Check sheet for the modelled part. Datum: model origin and axes. Units: mm. Give positions to 0.01 mm unless a question says otherwise; leave off trailing zeros. Loops run counter-clockwise (first coordinate to the right, second up) from the corner with the lowest first, then second, coordinate; pieces in that order, holes last. Notation, with made-up numbers: (51.5, 28.5) -> (77.5, 28.5) arc R17 cw to (77.5, 45.5) -> close; hole circle Ø8 at (-20.75, -0.75). An arc over 180 degrees is marked (long way). Write each question's results on one line, items separated by ' | '. Start each with the question number.
Item 1: Gauge pin test, flat ends, axial feed: pin 1 Ø1.5 at (y, z) = (-7, 5) entering from -X; pin 2 Ø3 at (y, z) = (17.5, 3.5) entering from +X. Record the tip position at first contact, or that the pin passes through.
Item 2: Cross-section at B-B on z = 12.25. Enter the section's corners in (x, y), then the cut area to 3 significant figures.
Item 3: Cross-section at C-C on z = 3.25. Enter the section's corners in (x, y).
Item 4: Scan lines: line 1 along X through (y, z) = (10.5, 2); line 2 along X through (y, z) = (-0.5, 3.25). Record each from-to range of solid material in increasing order.
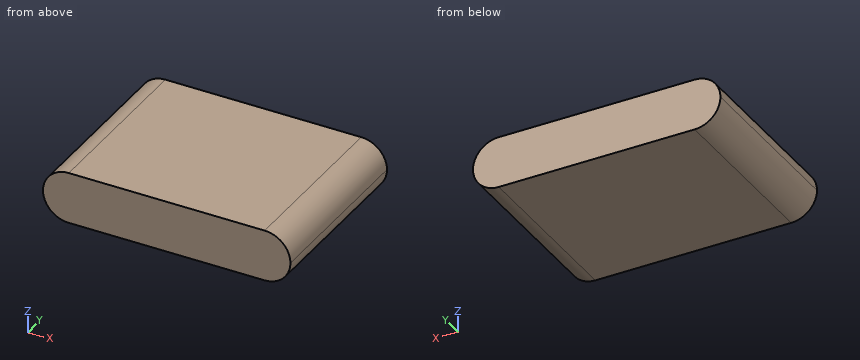
from build123d import *

# Parameters (mm, degrees)
SKETCH1_W           = 72
SKETCH1_H           = 51
BOSS_EXTRUDE1_DEPTH = 15
FILLET2_R           = 7.5
FILLET3_R           = 7.5


with BuildPart() as part:
    # Sketch1 → Boss-Extrude1 (new body)
    with BuildSketch(Plane.XY):
        Rectangle(SKETCH1_W, SKETCH1_H)
    extrude(amount=BOSS_EXTRUDE1_DEPTH)

    # Fillet2
    fillet2_edges = [part.edges().sort_by_distance(p)[0] for p in [
        (36, 0, 15),
    ]]
    fillet(fillet2_edges, radius=FILLET2_R)

    # Fillet3
    fillet3_edges = [part.edges().sort_by_distance(p)[0] for p in [
        (-36, 0, 15),
        (-36, 0, 0),
        (36, 0, 0),
    ]]
    fillet(fillet3_edges, radius=FILLET3_R - 0.0001)  # a hair under: the kernel refuses the full size


solid = part.part
Answer sheet:
1) pin 1: stops at x = -35.79 | pin 2: stops at x = 35.57
2) outline: (-34.3, -25.5) -> (34.3, -25.5) -> (34.3, 25.5) -> (-34.3, 25.5) -> close | area: 3,500 mm²
3) outline: (-34.68, -25.5) -> (34.68, -25.5) -> (34.68, 25.5) -> (-34.68, 25.5) -> close
4) line 1: x = -33.6 to 33.6 | line 2: x = -34.68 to 34.68
